from build123d import *

# Parameters (mm, degrees)
SKETCH_W        = 30
SKETCH_H        = 30
PAD_DEPTH       = 160
POCKET_DEPTH    = 30.001
SKETCH002_R     = 4
POCKET001_DEPTH = 113.138085
SKETCH003_R     = 12
POCKET002_DEPTH = 50
SKETCH004_R     = 3
POCKET003_DEPTH = 30.001


with BuildPart() as part:
    # Sketch → Pad (new body)
    with BuildSketch(Plane.XZ):
        with Locations((15, 15)):
            Rectangle(SKETCH_W, SKETCH_H)
    extrude(amount=PAD_DEPTH)

    # Sketch001 (on Face3 of Pad) → Pocket (cut, through all)
    with BuildSketch(Plane(origin=(0, 0, 30), x_dir=(-1, 0, 0), z_dir=(0, 0, 1))):
        Polygon((0, 0), (-30, 30), (-30, 0), align=None)
    extrude(amount=-POCKET_DEPTH, mode=Mode.SUBTRACT)

    # Sketch002 (on Face2 of Pocket) → Pocket001 (cut, through all)
    with BuildSketch(Plane(origin=(0, 0, 0), x_dir=(0.707107, -0.707107, 0), z_dir=(0.707107, 0.707107, 0))):
        with Locations((21.213203, -15)):
            Circle(SKETCH002_R)
    extrude(amount=-POCKET001_DEPTH, mode=Mode.SUBTRACT)

    # Sketch003 (on Face4 of Pocket001) → Pocket002 (cut)
    with BuildSketch(Plane.XZ.offset(160)):
        with Locations((15, 15)):
            Circle(SKETCH003_R)
    extrude(amount=-POCKET002_DEPTH, mode=Mode.SUBTRACT)

    # Sketch004 (on Face6 of Pocket002) → Pocket003 (cut, through all)
    with BuildSketch(Plane(origin=(0, 0, 30), x_dir=(-1, 0, 0), z_dir=(0, 0, 1))):
        with Locations((-15, 120)):
            Circle(SKETCH004_R)
    extrude(amount=-POCKET003_DEPTH, mode=Mode.SUBTRACT)


solid = part.part
Build history of the part. All positions in model axes, mm. A direction names the side the tool comes from. Give positions to 0.01 mm unless a question says otherwise; leave off trailing zeros. Order: outer loops, then holes, each group sorted by start corner. A loop starts at its lowest first (then second) coordinate and runs counter-clockwise, first axis right, second up. Notation, with made-up numbers: M -2.5,-30 L 31.5,-30 A22 cw 31.5,-16 Z; hole C -4,-27 d6. An arc over 180 degrees is marked long. Use one line per item in the form item = value.
Q1. Slice it at C-C, the plane z = 7.5. Write the cut outline in (x, y).
Conclusion:
outline = M 0,-160 L 5.63,-160 L 5.63,-110 L 24.37,-110 L 24.37,-160 L 30,-160 L 30,-30 L 0,0 Z
Q2. Wall check: probe 1 along Z at (x, y) = (15.5, -133.5); probe 2 along X at (y, z) = (-120, 29.2); probe 3 along X at (y, z) = (-126, 7.5). Give the ranges that are in metal, low to high.
Conclusion:
probe_1 = 0 to 3.01, 26.99 to 30
probe_2 = 0 to 12, 18 to 30
probe_3 = 0 to 5.63, 24.37 to 30
Q3. Pull direction X, two halves, no side cores. Call faces 1 (the flat face through (18, -18, 15)), 2 (the flat face through (0, -79, 15)), 3 (the cylindrical face through (26.446, -135.35, 18.604)): released by +X, released by -X, zero draft, split by the parting line, or undercut.
Conclusion:
face_1 = released by +X
face_2 = released by -X
face_3 = undercut
Q4. Slice it at D-D, the plane x = 15. State how many separate pieces and enclosed holes the cut face has, and give its area (3 significant figures).
Conclusion:
separate_pieces = 3
enclosed_holes = 0
area = 3,080 mm2
Q5. Slice it at A-A, the plane y = -120. Write the cut outline in (x, z).
Conclusion:
outline = M 0,0 L 12,0 L 12,3.38 A12 cw 12,26.62 L 12,30 L 0,30 Z; M 18,0 L 30,0 L 30,30 L 18,30 L 18,26.62 A12 cw 18,3.38 Z
Q6. Slice it at B-B, the plane z = 15. Write the cut outline in (x, y).
Conclusion:
outline = M 0,-160 L 3,-160 L 3,-110 L 27,-110 L 27,-160 L 30,-160 L 30,-30 L 17.83,-17.83 L 0,-35.66 Z; M 0,-24.34 L 12.17,-12.17 L 0,0 Z
Q7. Which spindle directions (+Z, -Z, +X, -X, +Y, -Y) get a long thin tool onto all of the face, cutting with end or side? Do faces 4 (the cylindrical face through (10.804, -24.421, 16.532)), 5 (the flat face through (15, -110, 15)). Say none if no direction does.
Conclusion:
face_4 = none
face_5 = -Y
Q8. Pin check, flat tips, straight feed: P1, Ø7, axis at x = 16.5, z = 12.5, coming from the -Y side; P2, Ø8, axis at x = 25, z = 22.5, coming from the +Y side. Stop position of each tip, or through.
Conclusion:
P1 = -110
P2 = -21
